The listing builds one solid part. Answer for the finished solid, in the listing's coordinates (mm). A direction names the side the tool comes from. Give positions to 0.01 mm unless a question says otherwise; leave off trailing zeros. Write each loop counter-clockwise with the first axis right and the second up, starting at its lowest first coordinate (ties: lowest second). Pieces come first, ordered by that corner, then holes.
```python
from build123d import *

# Parameters (mm, degrees)
SKETCH1_R           = 82
BOSS_EXTRUDE1_DEPTH = 7
SKETCH2_R           = 2.5
CUT_EXTRUDE1_DEPTH  = 10
SKETCH3_R           = 82
SKETCH3_R_2         = 78
BOSS_EXTRUDE2_DEPTH = 7
SKETCH4_R           = 1.25
CUT_EXTRUDE3_DEPTH  = 10
CIRPATTERN1_COUNT   = 4


with BuildPart() as part:
    # Sketch1 → Boss-Extrude1 (new body)
    with BuildSketch(Plane(origin=(0, 0, 0), x_dir=(1, 0, 0), z_dir=(0, 1, 0))):
        with Locations(Location((0, 0, 0), (0, 0, 270))):
            Circle(SKETCH1_R)
    extrude(amount=BOSS_EXTRUDE1_DEPTH)

    # Sketch2 → Cut-Extrude1 (cut)
    with BuildSketch(Plane(origin=(0, 7, 0), x_dir=(1, 0, 0), z_dir=(0, 1, 0))):
        with Locations(Location((-18.75, 0, 0), (0, 0, 270))):
            Circle(SKETCH2_R)
        with Locations(Location((18.75, 0, 0), (0, 0, 270))):
            Circle(SKETCH2_R)
    extrude(amount=-CUT_EXTRUDE1_DEPTH, mode=Mode.SUBTRACT)

    # Sketch3 → Boss-Extrude2 (add)
    with BuildSketch(Plane(origin=(0, 7, 0), x_dir=(1, 0, 0), z_dir=(0, 1, 0))):
        with Locations(Location((0, 0, 0), (0, 0, 270))):
            Circle(SKETCH3_R)
        with Locations(Location((0, 0, 0), (0, 0, 270))):
            Circle(SKETCH3_R_2, mode=Mode.SUBTRACT)
    extrude(amount=BOSS_EXTRUDE2_DEPTH)

    # Sketch4 → Cut-Extrude3 (cut)
    with BuildSketch(Plane(origin=(82, 0, 0), x_dir=(0, 0, -1), z_dir=(1, 0, 0))):
        with Locations((0, 7)):
            Circle(SKETCH4_R)
    cut_extrude3 = extrude(amount=-CUT_EXTRUDE3_DEPTH, mode=Mode.SUBTRACT)

    # CirPattern1: Cut-Extrude3 ×4 about axis
    cirpattern1_axis = Axis((0, 0, 0), (0, 1, 0))
    for i in range(1, CIRPATTERN1_COUNT):
        add(cut_extrude3.rotate(cirpattern1_axis, i * 360 / CIRPATTERN1_COUNT), mode=Mode.SUBTRACT)


solid = part.part
```
Item 1: Each of these flat-tipped pins is pushed along its axis until it touches: P1, Ø4, axis at y = 3.5, z = -19, coming from the -X side; P2, Ø1.5, axis at y = 6.5, z = -40, coming from the -X side; P3, Ø4, axis at x = -33.5, y = 4, coming from the +Z side. Where does it stop, or does it pass through?
Conclusion:
P1: stops at x = -80.22
P2: stops at x = -72
P3: stops at z = 75.71
Item 2: Which of the six approach directions +Z, -Z, +X, -X, +Y, -Y give full straight-line access (tool end or side, diameter ignored) to faces 1 (the face through (1, 0, -1)), 2 (the face through (77.336, 10.451, -10.154))?
Conclusion:
face 1: +Z, -Z, +X, -X, -Y
face 2: +Y
Item 3: Consider probe 1 along X at (y, z) = (5.5, 0); probe 2 along Z at (x, y) = (0, 10.25); probe 3 along Y at (x, z) = (61, -28.5). Determine where each line is inside the solid, lowest interval first.
Conclusion:
probe 1: x = -82 to -21.25, -16.25 to 16.25, 21.25 to 82
probe 2: z = -82 to -78, 78 to 82
probe 3: y = 0 to 7
Item 4: A cutting plane is placed at D-D, the plane x = -14. Give the vertices of the cut face in (y, z), plus the area to 3 significant figures.
Conclusion:
outline: (0, -80.8) - (14, -80.8) - (14, -76.73) - (7, -76.73) - (7, 76.73) - (14, 76.73) - (14, 80.8) - (0, 80.8) - close
area: 1,190 mm2
Item 5: A cutting plane is placed at A-A, the plane x = 18.75. Give the vertices of the cut face in (y, z).
Conclusion:
outline: (0, -79.83) - (14, -79.83) - (14, -75.71) - (7, -75.71) - (7, -2.5) - (0, -2.5) - close; (0, 2.5) - (7, 2.5) - (7, 75.71) - (14, 75.71) - (14, 79.83) - (0, 79.83) - close
Item 6: A cutting plane is placed at C-C, the plane y = 2.5. Give the vertices of the cut face in (x, z).
Conclusion:
outline: circle Ø164 at (0, 0); hole circle Ø5 at (-18.75, 0); hole circle Ø5 at (18.75, 0)
Item 7: Determine the mould class of faces 3 (the face through (-80, 7, -18)), 4 (the face through (-73, 14, 30)), 5 (the face through (-16.27, 3.55, -0.33)) for opening direction X: pulls with the +X half, pulls with the -X half, needs draft (parallel to the pull), parting line crosses it, or undercut.
Conclusion:
face 3: parting line crosses it
face 4: needs draft
face 5: undercut
Item 8: A cutting plane is placed at B-B, the plane z = 22. Give the vertices of the cut face in (x, y), plus the area to 3 significant figures.
Conclusion:
outline: (-78.99, 0) - (78.99, 0) - (78.99, 14) - (74.83, 14) - (74.83, 7) - (-74.83, 7) - (-74.83, 14) - (-78.99, 14) - close
area: 1,160 mm2
